Autodesk Inventor part; units mm, degrees
ref_plane "Work Plane2" through (0, 0, 7.9375) normal (0, 0, -1) x (-1, 0, 0)
ref_plane "YZ Plane" through (0, 0, 0) normal (1, 0, 0) x (0, 1, 0)
ref_plane "XZ Plane" through (0, 0, 0) normal (0, 1, 0) x (-1, 0, 0)
sketch "Sketch1" plane through (0, 0, 0) normal (0, 0, 1) x (1, 0, 0)
  circle A0 centre (0, 0) radius 2.5
  circle A1 centre (0, 0) radius 10
  dimension "d0" = 5
  dimension "d1" = 20
extrude "Extrusion1" add sketch "Sketch1" along normal blind 25
sketch "Sketch2" plane through (0, 0, 25) normal (0, 0, 1) x (1, 0, 0)
  circle A0 centre (0, 0) radius 2.5
  circle A1 centre (0, 0) radius 10
  circle A2 centre (0, 0) radius 4
  dimension "d4" = 8
extrude "Extrusion2" cut sketch "Sketch2" against normal blind 9.525 contours A2
ref_plane "Work Plane2" through (0, 0, 7.9375) normal (0, 0, -1) x (-1, 0, 0)
sketch "Sketch6" plane through (0, 0, 7.9375) normal (0, 0, -1) x (-1, 0, 0)
  circle A0 centre (0, 0) radius 11
  circle A1 centre (0, 0) radius 9.5
  dimension "d11" = 22
  dimension "d14" = 19
extrude "Extrusion5" cut sketch "Sketch6" against normal blind 2
pattern_linear "Rectangular Pattern1" count 3 spacing 4 along (0, 0, 1) of "Extrusion5"
properties part number "SM-H12"
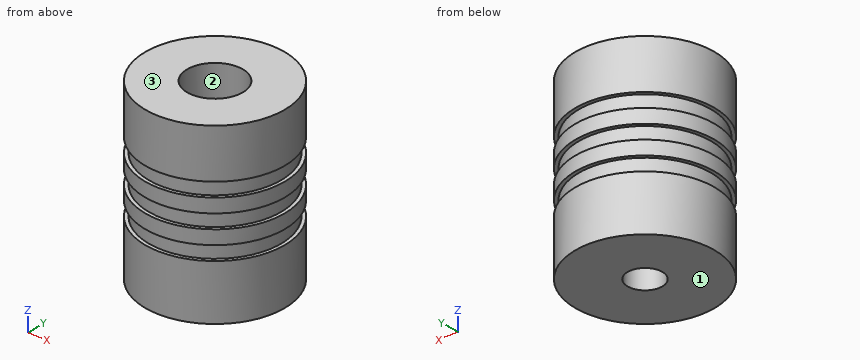
Part model, mm, in its own coordinate system. Face numbers are marked on the shaded views. Give positions to 0.01 mm unless a question says otherwise; leave off trailing zeros. Write each loop counter-clockwise with the first axis right and the second up, starting at its lowest first coordinate (ties: lowest second). Pieces come first, ordered by that corner, then holes.
1) Cut at D-D on z = 17. Write the cut outline in (x, y), then the cut area to 3 significant figures.
Resolved:
outline: circle Ø19 at (0, 0); hole circle Ø8 at (0, 0)
area: 233 mm2
2) Probe L1, parallel to Z at x = 5.5, y = 8.25; L2, parallel to Y at x = 0, z = 5.5; L3, parallel to X at y = -1.5, z = 4. List the from-to ranges inside material, lowest first.
Resolved:
L1: z = 0 to 7.94, 9.94 to 11.94, 13.94 to 15.94, 17.94 to 25
L2: y = -10 to -2.5, 2.5 to 10
L3: x = -9.89 to -2, 2 to 9.89
3) Cut at A-A on z = 8.75. Write the cut outline in (x, y), then the cut area to 3 significant figures.
Resolved:
outline: circle Ø19 at (0, 0); hole circle Ø5 at (0, 0)
area: 264 mm2
4) Pin check, flat tips, straight feed: pin 1 (5 mm diameter, centred on y = -3, z = 4, fed in from -X); pin 2 (4 mm diameter, centred on y = -2.5, z = 13, fed in from +X); pin 3 (2 mm diameter, centred on x = 2.5, z = 10, fed in from +Y). Stop position of each tip, or through.
Resolved:
pin 1: stops at x = -9.99
pin 2: stops at x = 9.97
pin 3: stops at y = 9.89
5) Two-plate mould, pull along Z, no slides. Class the marked faces 1, 2 and 3: released by +Z, released by -Z, zero draft, split by the parting line, or undercut.
Resolved:
face 1: released by -Z
face 2: zero draft
face 3: released by +Z
6) Cut at B-B on x = 7.5. Write the cut outline in (y, z).
Resolved:
outline: (-6.61, 0) - (6.61, 0) - (6.61, 7.94) - (5.83, 7.94) - (5.83, 9.94) - (6.61, 9.94) - (6.61, 11.94) - (5.83, 11.94) - (5.83, 13.94) - (6.61, 13.94) - (6.61, 15.94) - (5.83, 15.94) - (5.83, 17.94) - (6.61, 17.94) - (6.61, 25) - (-6.61, 25) - (-6.61, 17.94) - (-5.83, 17.94) - (-5.83, 15.94) - (-6.61, 15.94) - (-6.61, 13.94) - (-5.83, 13.94) - (-5.83, 11.94) - (-6.61, 11.94) - (-6.61, 9.94) - (-5.83, 9.94) - (-5.83, 7.94) - (-6.61, 7.94) - close
7) Cut at C-C on y = 5.5. Write the cut outline in (x, z).
Resolved:
outline: (-8.35, 0) - (8.35, 0) - (8.35, 7.94) - (7.75, 7.94) - (7.75, 9.94) - (8.35, 9.94) - (8.35, 11.94) - (7.75, 11.94) - (7.75, 13.94) - (8.35, 13.94) - (8.35, 15.94) - (7.75, 15.94) - (7.75, 17.94) - (8.35, 17.94) - (8.35, 25) - (-8.35, 25) - (-8.35, 17.94) - (-7.75, 17.94) - (-7.75, 15.94) - (-8.35, 15.94) - (-8.35, 13.94) - (-7.75, 13.94) - (-7.75, 11.94) - (-8.35, 11.94) - (-8.35, 9.94) - (-7.75, 9.94) - (-7.75, 7.94) - (-8.35, 7.94) - close
